```python
from build123d import *

# Parameters (mm, degrees)
F0_R     = 10
F1_DEPTH = 25
F2_R     = 5
F3_DEPTH = 12.5
F4_R     = 3.175
F5_DEPTH = 25.001


with BuildPart() as f1:
    # F0 (on Front) → F1 (new body)
    with BuildSketch(Plane.XZ):
        Circle(F0_R)
    extrude(amount=F1_DEPTH)

    # F2 (on face) → F3 (cut)
    with BuildSketch(Plane.XZ.offset(25)):
        Circle(F2_R)
    extrude(amount=-F3_DEPTH, mode=Mode.SUBTRACT)

    # F4 (on face) → F5 (cut, through all)
    with BuildSketch(Plane(origin=(0, 0, 0), x_dir=(-1, 0, 0), z_dir=(0, 1, 0))):
        Circle(F4_R)
    extrude(amount=-F5_DEPTH, mode=Mode.SUBTRACT)


solid = f1.part
```
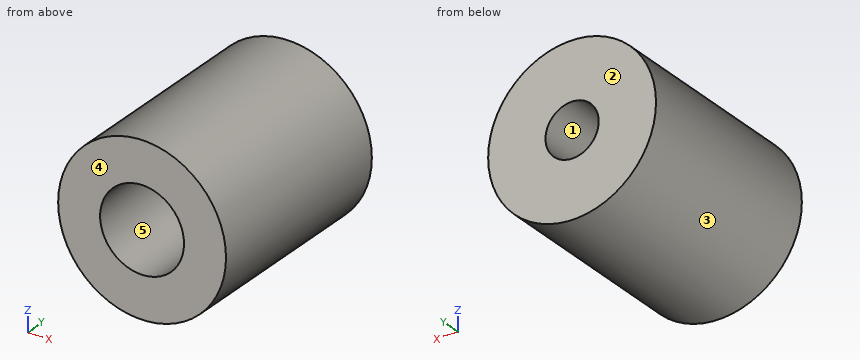
The model under review builds one solid part; all positions refer to its coordinate system, in mm. Face numbers are marked on the shaded views. A direction names the side the tool comes from. Give positions to 0.01 mm unless a question says otherwise; leave off trailing zeros. Write each loop counter-clockwise with the first axis right and the second up, starting at its lowest first coordinate (ties: lowest second). Pieces come first, ordered by that corner, then holes. Notation, with made-up numbers: M 53.5,13.5 L 78.5,13.5 A14 ccw 78.5,38.5 Z; hole C 77.25,-1.75 d6. An arc over 180 degrees is marked long. Write item = value, one per line. Start each with the question number.
Q1. Clearance check with flat-ended pins moving along their axes: pin 1 (1.5 mm diameter, centred on x = -4.5, y = -8.5, fed in from -Z); pin 2 (10 mm diameter, centred on y = -17, z = 6, fed in from +X); pin 3 (4 mm diameter, centred on x = 0, z = 0, fed in from +Y); pin 4 (5 mm diameter, centred on x = 6.5, y = -17, fed in from +Z). State where each tip first meets the part, or that it passes through.
Q2. We need section C-C (y = -13.5). State the section outline as (x, z) points.
Q3. Machinability: for the marked faces 4 and 5, which of the approach directions +Z, -Z, +X, -X, +Y, -Y give a long, thin tool a straight path to every point of the face, cutting with its end or side? Answer none if there is none.
Q4. We need section A-A (z = 0). State the section outline as (x, y) points (3 decimals).
Q5. For line 1 (Z direction, x = 0, y = -18); line 2 (Z direction, x = 1.5, y = -20); line 3 (X direction, y = -17.5, z = -1.75), list the stretches that pass through material, from the lowest coordinate up.
Q6. Mouldability with a two-part tool opening along Z and no side actions: class the marked faces 1, 2 and 3 as released by +Z, released by -Z, zero draft, split by the parting line, or undercut.
Q7. We need section D-D (x = 8). State the section outline as (y, z) points, plus the area to 3 significant figures.
Q8. We need section B-B (x = 0). State the section outline as (y, z) points (3 decimals).
Result set:
q1.pin_1 = -9.27
q1.pin_2 = 9.95
q1.pin_3 = through
q1.pin_4 = 9.17
q2.outline = C 0,0 d20; hole C 0,0 d10
q3.face_4 = +Z, -Z, +X, -X, -Y
q3.face_5 = -Y
q4.outline = M -10,-25 L -5,-25 L -5,-12.5 L -3.175,-12.5 L -3.175,0 L -10,0 Z; M 3.175,-12.5 L 5,-12.5 L 5,-25 L 10,-25 L 10,0 L 3.175,0 Z
q5.line_1 = -10 to -5, 5 to 10
q5.line_2 = -9.89 to -4.77, 4.77 to 9.89
q5.line_3 = -9.85 to -4.68, 4.68 to 9.85
q6.face_1 = undercut
q6.face_2 = zero draft
q6.face_3 = split by the parting line
q7.outline = M -25,-6 L 0,-6 L 0,6 L -25,6 Z
q7.area = 300 mm2
q8.outline = M -25,-10 L 0,-10 L 0,-3.175 L -12.5,-3.175 L -12.5,-5 L -25,-5 Z; M -25,5 L -12.5,5 L -12.5,3.175 L 0,3.175 L 0,10 L -25,10 Z
